from build123d import *

# Parameters (mm, degrees)
SKETCH010_W     = 98
SKETCH010_H     = 59
PAD007_DEPTH    = 25
SKETCH011_W     = 95
SKETCH011_H     = 56
POCKET002_DEPTH = 22
SKETCH012_W     = 56
SKETCH012_H     = 2
PAD008_DEPTH    = 1
SKETCH013_W     = 56.025157
SKETCH013_H     = 2
PAD009_DEPTH    = 1
POCKET003_DEPTH = 53
SKETCH017_R     = 0.869454
SKETCH017_R_2   = 0.804164
PAD010_DEPTH    = 1


with BuildPart() as part:
    # Sketch010 → Pad007 (new body)
    with BuildSketch(Plane.XY):
        Rectangle(SKETCH010_W, SKETCH010_H)
    extrude(amount=PAD007_DEPTH)

    # Sketch011 (on Face6 of Pad007) → Pocket002 (cut)
    with BuildSketch(Plane.XY.offset(25)):
        Rectangle(SKETCH011_W, SKETCH011_H)
    extrude(amount=-POCKET002_DEPTH, mode=Mode.SUBTRACT)

    # Sketch012 (on Face9 of Pocket002) → Pad008 (join)
    with BuildSketch(Plane.YZ.offset(-47.5)):
        with Locations((0, 14.5)):
            Rectangle(SKETCH012_W, SKETCH012_H)
    extrude(amount=PAD008_DEPTH)

    # Sketch013 (on Face7 of Pad008) → Pad009 (join)
    with BuildSketch(Plane(origin=(47.5, 0, 0), x_dir=(0, -1, 0), z_dir=(-1, 0, 0))):
        with Locations((0.0125785, 14.5)):
            Rectangle(SKETCH013_W, SKETCH013_H)
    extrude(amount=PAD009_DEPTH)

    # Sketch015 (on Face1 of Pad009) → Pocket003 (cut)
    with BuildSketch(Plane.YZ.offset(49)):
        Polygon((-27.5, 1.5), (-26.75, 5), (-5.75, 5), (-5, 1.5), align=None)
    extrude(amount=-POCKET003_DEPTH, mode=Mode.SUBTRACT)

    # Sketch017 (on Face9 of Pocket003) → Pad010 (join)
    with BuildSketch(Plane.XY.offset(1.5)):
        with Locations((-2.011455, -10.80103)):
            Circle(SKETCH017_R)
        with Locations((-2.011455, -22.201292)):
            Circle(SKETCH017_R_2)
    extrude(amount=PAD010_DEPTH)


solid = part.part
Geometry: final body of the model. Coordinates: model frame, mm. A direction names the side the tool comes from. Give positions to 0.01 mm unless a question says otherwise; leave off trailing zeros. Write each loop counter-clockwise with the first axis right and the second up, starting at its lowest first coordinate (ties: lowest second). Pieces come first, ordered by that corner, then holes. Notation, with made-up numbers: M 41,4.5 L 53,4.5 A29 cw 53,42.5 Z; hole C -4,-26.5 d5. An arc over 180 degrees is marked long. Answer in a Markdown table with one row per item. Add a question column.
(1) Section B-B on z = 7.25. Return loops of the section in (x, y), and give its area (3 significant figures).
(2) Reachability of faces 4 (the flat face through (46.5, 0, 15)), 5 (the flat face through (22.871, -5.214, 2.497)), 6 (the flat face through (-47.5, 0, 8)) from +Z, -Z, +X, -X, +Y, -Y: full face, straight path, thin tool, end or side. Return the list, or none.
(3) First-contact query: pin 1 (1.4 mm diameter, centred on x = -2, y = -11, fed in from +Z); pin 2 (0.8 mm diameter, centred on x = 47, y = 1.5, fed in from +Z); pin 3 (10 mm diameter, centred on x = -2, y = -12, fed in from +Z). Flat tips, straight axial feed; report the tip coordinate or a pass-through.
(4) Section C-C on x = -10.5. Return loops of the section in (y, z).
(5) Section A-A on y = -24. Return loops of the section in (x, z).
(6) Mould query, pull axis Y, two halves, no side actions, for faces 1 (the flat face through (47.5, 0, 8)), 2 (the flat face through (-1, -29.5, 12)), 3 (the flat face through (0, 29, 25)). Classes: +Y half, -Y half, draft (parallel to the pull), parting line (faces both ways), or undercut.
(7) Ray query, line 1 (X direction, y = 4, z = 5.5); line 2 (Y direction, x = -36, z = 10.5); line 3 (Z direction, x = -38.5, y = -2). Return the intervals inside material, ascending.
(8) Section D-D on y = 13. Return loops of the section in (x, z), and give its area (3 significant figures).
Result set:
| question | item | result |
|---|---|---|
| 1 | outline | M -49,-29.5 L 49,-29.5 L 49,29.5 L -49,29.5 Z; hole M -47.5,-28 L 47.5,-28 L 47.5,28 L -47.5,28 Z |
| 1 | area | 462 mm^2 |
| 2 | face 4 | +Z |
| 2 | face 5 | +X |
| 2 | face 6 | none |
| 3 | pin 1 | stops at z = 2.5 |
| 3 | pin 2 | stops at z = 15.5 |
| 3 | pin 3 | stops at z = 3 |
| 4 | outline | M -29.5,0 L 29.5,0 L 29.5,25 L 28,25 L 28,3 L -28,3 L -28,25 L -29.5,25 Z |
| 5 | outline | M -49,0 L 49,0 L 49,1.5 L -4,1.5 L -4,3 L -47.5,3 L -47.5,13.5 L -46.5,13.5 L -46.5,15.5 L -47.5,15.5 L -47.5,25 L -49,25 Z; M 46.5,13.5 L 47.5,13.5 L 47.5,5 L 49,5 L 49,25 L 47.5,25 L 47.5,15.5 L 46.5,15.5 Z |
| 6 | face 1 | undercut |
| 6 | face 2 | -Y half |
| 6 | face 3 | draft |
| 7 | line 1 | x = -49 to -47.5, 47.5 to 49 |
| 7 | line 2 | y = -29.5 to -28, 28 to 29.5 |
| 7 | line 3 | z = 0 to 3 |
| 8 | outline | M -49,0 L 49,0 L 49,25 L 47.5,25 L 47.5,15.5 L 46.5,15.5 L 46.5,13.5 L 47.5,13.5 L 47.5,3 L -47.5,3 L -47.5,13.5 L -46.5,13.5 L -46.5,15.5 L -47.5,15.5 L -47.5,25 L -49,25 Z |
| 8 | area | 364 mm^2 |
